```python
from build123d import *

# Parameters (mm, degrees)
BOSS_EXTRUDE1_DEPTH   = 12.7
BOSS_EXTRUDE2_DEPTH   = 152.4
F_6_32_TAPPED_HOLE1_D = 3.400000058
CHAMFER1_SIZE         = 0.5


with BuildPart() as part:
    # Sketch2 → Boss-Extrude1 (new body)
    with BuildSketch(Plane.XY):
        Polygon((-76.2, 5.08), (-81.28, 0), (-76.2, -5.08), (-76.2, -10.16), (76.2, -10.16), (76.2, -5.08), (81.28, 0), (76.2, 5.08), (76.2, 10.16), (-76.2, 10.16), align=None)
    extrude(amount=BOSS_EXTRUDE1_DEPTH)

    # Sketch3 → Boss-Extrude2 (add)
    with BuildSketch(Plane.XY.offset(12.7)):
        Polygon((-76.2, 10.16), (-63.5, 10.16), (-63.5, 5.08), (-58.42, 0), (-63.5, -5.08), (-63.5, -10.16), (-76.2, -10.16), (-76.2, -5.08), (-81.28, 0), (-76.2, 5.08), align=None)
        Polygon((63.5, 10.16), (63.5, 5.08), (58.42, 0), (63.5, -5.08), (63.5, -10.16), (76.2, -10.16), (76.2, -5.08), (81.28, 0), (76.2, 5.08), (76.2, 10.16), align=None)
    extrude(amount=BOSS_EXTRUDE2_DEPTH)

    # #6-32 Tapped Hole1 (through all)
    with Locations(Plane.XY.offset(165.1)):
        with Locations((-69.85, 6.35), (-69.85, -6.35), (69.85, 6.35), (69.85, -6.35)):
            Hole(F_6_32_TAPPED_HOLE1_D / 2)

    # Chamfer1
    chamfer1_edges = [part.edges().sort_by_distance(p)[0] for p in [
        (0, -10.16, 0),
        (0, 10.16, 0),
        (76.2, -10.16, 82.55),
        (-76.2, -10.16, 82.55),
        (-76.2, 10.16, 82.55),
        (76.2, 10.16, 82.55),
        (0, -10.16, 12.7),
        (-63.5, -10.16, 88.9),
        (-63.5, 10.16, 88.9),
        (-69.85, -10.16, 165.1),
        (-69.85, 10.16, 165.1),
        (0, 10.16, 12.7),
        (63.5, 10.16, 88.9),
        (63.5, -10.16, 88.9),
        (69.85, 10.16, 165.1),
        (69.85, -10.16, 165.1),
    ]]
    chamfer(chamfer1_edges, length=CHAMFER1_SIZE)


solid = part.part
```
The model under review builds one solid part; all positions refer to its coordinate system, in mm. A direction names the side the tool comes from. Give positions to 0.01 mm unless a question says otherwise; leave off trailing zeros. Write each loop counter-clockwise with the first axis right and the second up, starting at its lowest first coordinate (ties: lowest second). Pieces come first, ordered by that corner, then holes.
(1) The part is to be moulded in two halves that separate along X. For faces 1 (the flat face through (-63.5, -7, 88)), 2 (the flat face through (76.2, 7, 81)), 3 (the flat face through (-12, 10.16, 9)), say which applies: released by +X, released by -X, zero draft, split by the parting line, or undercut.
(2) To check wall thickness, follow L1, parallel to X at y = -6.25, z = 154; L2, parallel to Y at x = -69.85, z = 58.5; L3, parallel to Y at x = -68.5, z = 157.5. State the ranges of each line that lie inside material, in increasing order.
(3) For P1, Ø2.5, axis at y = 8, z = 86.5, coming from the +X side; P2, Ø2.5, axis at x = 69.85, y = 6.35, coming from the -Z side; P3, Ø5, axis at y = -6.5, z = 123, coming from the -X side; P4, Ø5, axis at x = -51, y = -6.5, coming from the +Z side, all flat-tipped, find the tip position at first contact; note any pin that passes through.
(4) Consider section A-A, the plane z = 18.5. Give the number of separate pieces and of enclosed holes in the cut face, and give its area (3 significant figures).
(5) Consider section B-B, the plane x = -21. Give the boundary of the cut face in (y, z).
(6) Tool access review of faces 4 (the flat face through (63.5, 7, 88)), 5 (the flat face through (76.2, -7, 81)), 6 (the flat face through (-76.2, 7, 81)): name each direction out of +Z, -Z, +X, -X, +Y, -Y from which nothing blocks a thin tool from reaching the whole face with its end or side.
Returned:
1. face 1: undercut
1. face 2: released by +X
1. face 3: zero draft
2. L1: x = -76.2 to -71.55, -68.15 to -63.5, 63.5 to 68.15, 71.55 to 76.2
2. L2: y = -10.16 to -8.05, -4.65 to 4.65, 8.05 to 10.16
2. L3: y = -10.16 to -7.38, -5.32 to 5.32, 7.38 to 10.16
3. P1: stops at x = 76.2
3. P2: passes through
3. P3: stops at x = -77.28
3. P4: stops at z = 12.7
4. separate pieces: 2
4. enclosed holes: 4
4. area: 582 mm2
5. outline: (-10.16, 0.5) - (-9.66, 0) - (9.66, 0) - (10.16, 0.5) - (10.16, 12.2) - (9.66, 12.7) - (-9.66, 12.7) - (-10.16, 12.2) - close
6. face 4: +Z, +Y
6. face 5: +Z, -Z, +X, -Y
6. face 6: +Z, -Z, -X, +Y
